from build123d import *
from OCP.BRepFilletAPI import BRepFilletAPI_MakeChamfer

# Parameters (mm, degrees)
SKETCH1_W                     = 2.54
SKETCH1_H                     = 2.54
MAIN_BODY_DEPTH               = 2.54
SKETCH3_W                     = 1.778
SKETCH3_H                     = 0.381
CUT_EXTRUDE1_DEPTH            = 5.399409051
CUT_EXTRUDE2_DEPTH            = 5.399409051
BODY_PATTERN_COUNT            = 4
BODY_PATTERN_PITCH            = 2.54
PIN_START                     = -5.54
SKETCH2_W                     = 0.64
SKETCH2_H                     = 0.64
PIN_DEPTH                     = 11.54
CHAMFER1_SIZE                 = 0.508
CHAMFER1_SIZE2                = 0.1905
CHAMFER2_SIZE                 = 0.1905
CHAMFER2_SIZE2                = 0.508
PIN_PATTERN_COUNT             = 4
PIN_PATTERN_PITCH             = 2.54
CHAMFER1_OF_PIN_PATTERN_SIZE  = 0.508
CHAMFER1_OF_PIN_PATTERN_SIZE2 = 0.1905
CHAMFER2_OF_PIN_PATTERN_SIZE2 = 0.1905
CHAMFER2_OF_PIN_PATTERN_SIZE  = 0.508


with BuildPart() as part:
    # Sketch1 → Main Body (new body)
    with BuildSketch(Plane(origin=(0, 0, 0), x_dir=(1, 0, 0), z_dir=(0, 1, 0))):
        with Locations((1.27, 1.27)):
            Rectangle(SKETCH1_W, SKETCH1_H)
    main_body = extrude(amount=MAIN_BODY_DEPTH)

    # Sketch3 → Cut-Extrude1 (cut, through all)
    with BuildSketch(Plane.ZY):
        with Locations((-1.27, 0.1905)):
            Rectangle(SKETCH3_W, SKETCH3_H)
    cut_extrude1 = extrude(amount=-CUT_EXTRUDE1_DEPTH, mode=Mode.SUBTRACT)

    # Sketch4 → Cut-Extrude2 (cut, through all)
    with BuildSketch(Plane(origin=(0, 2.54, 0), x_dir=(1, 0, 0), z_dir=(0, 1, 0))):
        Polygon((0.254, 2.54), (0, 2.54), (0, 2.032), align=None)
        Polygon((2.54, 2.54), (2.286, 2.54), (2.54, 2.032), align=None)
        Polygon((0.254, 0), (0, 0.508), (0, 0), align=None)
        Polygon((2.54, 0), (2.286, 0), (2.54, 0.508), align=None)
    cut_extrude2 = extrude(amount=-CUT_EXTRUDE2_DEPTH, mode=Mode.SUBTRACT)

    # Body Pattern: Main Body, Cut-Extrude1, Cut-Extrude2 ×4
    with Locations(*[(-i * BODY_PATTERN_PITCH, 0, 0) for i in range(1, BODY_PATTERN_COUNT)]):
        add(main_body)
        add(cut_extrude1, mode=Mode.SUBTRACT)
        add(cut_extrude2, mode=Mode.SUBTRACT)

    # Sketch2 → Pin (add)
    with BuildSketch(Plane(origin=(0, 2.54, 0), x_dir=(1, 0, 0), z_dir=(0, 1, 0)).offset(PIN_START)):
        with Locations((1.27, 1.27)):
            Rectangle(SKETCH2_W, SKETCH2_H)
    pin = extrude(amount=PIN_DEPTH)

    # Chamfer1: one chamfer whose edges measure the first distance from different faces: ONE call of the kernel's chamfer builder (chamfer() names one face for all edges)
    chamfer1_edges_1 = [part.edges().sort_by_distance(p)[0] for p in [
        (0.95, 8.54, -1.27),
    ]]
    chamfer1_side_1 = [part.faces().sort_by_distance(p)[0] for p in [
        (0.95, 5.54, -1.27),
    ]]
    chamfer1_edges_2 = [part.edges().sort_by_distance(p)[0] for p in [
        (1.27, 8.54, -0.95),
    ]]
    chamfer1_side_2 = [part.faces().sort_by_distance(p)[0] for p in [
        (1.27, 5.54, -0.95),
    ]]
    chamfer1_edges_3 = [part.edges().sort_by_distance(p)[0] for p in [
        (1.59, 8.54, -1.27),
    ]]
    chamfer1_side_3 = [part.faces().sort_by_distance(p)[0] for p in [
        (1.59, 5.54, -1.27),
    ]]
    chamfer1_edges_4 = [part.edges().sort_by_distance(p)[0] for p in [
        (1.27, 8.54, -1.59),
    ]]
    chamfer1_side_4 = [part.faces().sort_by_distance(p)[0] for p in [
        (1.27, 5.54, -1.59),
    ]]
    chamfer1 = BRepFilletAPI_MakeChamfer(part.part.solid().wrapped)
    for e in chamfer1_edges_1:
        chamfer1.Add(CHAMFER1_SIZE, CHAMFER1_SIZE2, e.wrapped, chamfer1_side_1[0].wrapped)  # the first distance lies on this face
    for e in chamfer1_edges_2:
        chamfer1.Add(CHAMFER1_SIZE, CHAMFER1_SIZE2, e.wrapped, chamfer1_side_2[0].wrapped)  # the first distance lies on this face
    for e in chamfer1_edges_3:
        chamfer1.Add(CHAMFER1_SIZE, CHAMFER1_SIZE2, e.wrapped, chamfer1_side_3[0].wrapped)  # the first distance lies on this face
    for e in chamfer1_edges_4:
        chamfer1.Add(CHAMFER1_SIZE, CHAMFER1_SIZE2, e.wrapped, chamfer1_side_4[0].wrapped)  # the first distance lies on this face
    add(Compound.cast(chamfer1.Shape()), mode=Mode.REPLACE)

    # Chamfer2
    chamfer2_edges = [part.edges().sort_by_distance(p)[0] for p in [
        (1.27, -3, -0.95),
        (1.59, -3, -1.27),
        (1.27, -3, -1.59),
        (0.95, -3, -1.27),
    ]]
    chamfer2_side = [part.faces().sort_by_distance(p)[0] for p in [
        (1.27, -3, -1.27),
    ]]
    chamfer(chamfer2_edges, length=CHAMFER2_SIZE, length2=CHAMFER2_SIZE2, reference=chamfer2_side[0])

    # Pin Pattern: Pin ×4
    with Locations(*[(-i * PIN_PATTERN_PITCH, 0, 0) for i in range(1, PIN_PATTERN_COUNT)]):
        add(pin)

    # Chamfer1 of Pin Pattern: one chamfer whose edges measure the first distance from different faces: ONE call of the kernel's chamfer builder (chamfer() names one face for all edges)
    chamfer1_of_pin_pattern_edges_1 = [part.edges().sort_by_distance(p)[0] for p in [
        (-1.59, 8.54, -1.27),
    ]]
    chamfer1_of_pin_pattern_side_1 = [part.faces().sort_by_distance(p)[0] for p in [
        (-1.59, 5.54, -1.27),
    ]]
    chamfer1_of_pin_pattern_edges_2 = [part.edges().sort_by_distance(p)[0] for p in [
        (-1.27, 8.54, -0.95),
    ]]
    chamfer1_of_pin_pattern_side_2 = [part.faces().sort_by_distance(p)[0] for p in [
        (-1.27, 5.54, -0.95),
    ]]
    chamfer1_of_pin_pattern_edges_3 = [part.edges().sort_by_distance(p)[0] for p in [
        (-0.95, 8.54, -1.27),
    ]]
    chamfer1_of_pin_pattern_side_3 = [part.faces().sort_by_distance(p)[0] for p in [
        (-0.95, 5.54, -1.27),
    ]]
    chamfer1_of_pin_pattern_edges_4 = [part.edges().sort_by_distance(p)[0] for p in [
        (-1.27, 8.54, -1.59),
    ]]
    chamfer1_of_pin_pattern_side_4 = [part.faces().sort_by_distance(p)[0] for p in [
        (-1.27, 5.54, -1.59),
    ]]
    chamfer1_of_pin_pattern_edges_5 = [part.edges().sort_by_distance(p)[0] for p in [
        (-4.13, 8.54, -1.27),
    ]]
    chamfer1_of_pin_pattern_side_5 = [part.faces().sort_by_distance(p)[0] for p in [
        (-4.13, 5.54, -1.27),
    ]]
    chamfer1_of_pin_pattern_edges_6 = [part.edges().sort_by_distance(p)[0] for p in [
        (-3.81, 8.54, -0.95),
    ]]
    chamfer1_of_pin_pattern_side_6 = [part.faces().sort_by_distance(p)[0] for p in [
        (-3.81, 5.54, -0.95),
    ]]
    chamfer1_of_pin_pattern_edges_7 = [part.edges().sort_by_distance(p)[0] for p in [
        (-3.49, 8.54, -1.27),
    ]]
    chamfer1_of_pin_pattern_side_7 = [part.faces().sort_by_distance(p)[0] for p in [
        (-3.49, 5.54, -1.27),
    ]]
    chamfer1_of_pin_pattern_edges_8 = [part.edges().sort_by_distance(p)[0] for p in [
        (-3.81, 8.54, -1.59),
    ]]
    chamfer1_of_pin_pattern_side_8 = [part.faces().sort_by_distance(p)[0] for p in [
        (-3.81, 5.54, -1.59),
    ]]
    chamfer1_of_pin_pattern_edges_9 = [part.edges().sort_by_distance(p)[0] for p in [
        (-6.67, 8.54, -1.27),
    ]]
    chamfer1_of_pin_pattern_side_9 = [part.faces().sort_by_distance(p)[0] for p in [
        (-6.67, 5.54, -1.27),
    ]]
    chamfer1_of_pin_pattern_edges_10 = [part.edges().sort_by_distance(p)[0] for p in [
        (-6.35, 8.54, -0.95),
    ]]
    chamfer1_of_pin_pattern_side_10 = [part.faces().sort_by_distance(p)[0] for p in [
        (-6.35, 5.54, -0.95),
    ]]
    chamfer1_of_pin_pattern_edges_11 = [part.edges().sort_by_distance(p)[0] for p in [
        (-6.03, 8.54, -1.27),
    ]]
    chamfer1_of_pin_pattern_side_11 = [part.faces().sort_by_distance(p)[0] for p in [
        (-6.03, 5.54, -1.27),
    ]]
    chamfer1_of_pin_pattern_edges_12 = [part.edges().sort_by_distance(p)[0] for p in [
        (-6.35, 8.54, -1.59),
    ]]
    chamfer1_of_pin_pattern_side_12 = [part.faces().sort_by_distance(p)[0] for p in [
        (-6.35, 5.54, -1.59),
    ]]
    chamfer1_of_pin_pattern = BRepFilletAPI_MakeChamfer(part.part.solid().wrapped)
    for e in chamfer1_of_pin_pattern_edges_1:
        chamfer1_of_pin_pattern.Add(CHAMFER1_OF_PIN_PATTERN_SIZE, CHAMFER1_OF_PIN_PATTERN_SIZE2, e.wrapped, chamfer1_of_pin_pattern_side_1[0].wrapped)  # the first distance lies on this face
    for e in chamfer1_of_pin_pattern_edges_2:
        chamfer1_of_pin_pattern.Add(CHAMFER1_OF_PIN_PATTERN_SIZE, CHAMFER1_OF_PIN_PATTERN_SIZE2, e.wrapped, chamfer1_of_pin_pattern_side_2[0].wrapped)  # the first distance lies on this face
    for e in chamfer1_of_pin_pattern_edges_3:
        chamfer1_of_pin_pattern.Add(CHAMFER1_OF_PIN_PATTERN_SIZE, CHAMFER1_OF_PIN_PATTERN_SIZE2, e.wrapped, chamfer1_of_pin_pattern_side_3[0].wrapped)  # the first distance lies on this face
    for e in chamfer1_of_pin_pattern_edges_4:
        chamfer1_of_pin_pattern.Add(CHAMFER1_OF_PIN_PATTERN_SIZE, CHAMFER1_OF_PIN_PATTERN_SIZE2, e.wrapped, chamfer1_of_pin_pattern_side_4[0].wrapped)  # the first distance lies on this face
    for e in chamfer1_of_pin_pattern_edges_5:
        chamfer1_of_pin_pattern.Add(CHAMFER1_OF_PIN_PATTERN_SIZE, CHAMFER1_OF_PIN_PATTERN_SIZE2, e.wrapped, chamfer1_of_pin_pattern_side_5[0].wrapped)  # the first distance lies on this face
    for e in chamfer1_of_pin_pattern_edges_6:
        chamfer1_of_pin_pattern.Add(CHAMFER1_OF_PIN_PATTERN_SIZE, CHAMFER1_OF_PIN_PATTERN_SIZE2, e.wrapped, chamfer1_of_pin_pattern_side_6[0].wrapped)  # the first distance lies on this face
    for e in chamfer1_of_pin_pattern_edges_7:
        chamfer1_of_pin_pattern.Add(CHAMFER1_OF_PIN_PATTERN_SIZE, CHAMFER1_OF_PIN_PATTERN_SIZE2, e.wrapped, chamfer1_of_pin_pattern_side_7[0].wrapped)  # the first distance lies on this face
    for e in chamfer1_of_pin_pattern_edges_8:
        chamfer1_of_pin_pattern.Add(CHAMFER1_OF_PIN_PATTERN_SIZE, CHAMFER1_OF_PIN_PATTERN_SIZE2, e.wrapped, chamfer1_of_pin_pattern_side_8[0].wrapped)  # the first distance lies on this face
    for e in chamfer1_of_pin_pattern_edges_9:
        chamfer1_of_pin_pattern.Add(CHAMFER1_OF_PIN_PATTERN_SIZE, CHAMFER1_OF_PIN_PATTERN_SIZE2, e.wrapped, chamfer1_of_pin_pattern_side_9[0].wrapped)  # the first distance lies on this face
    for e in chamfer1_of_pin_pattern_edges_10:
        chamfer1_of_pin_pattern.Add(CHAMFER1_OF_PIN_PATTERN_SIZE, CHAMFER1_OF_PIN_PATTERN_SIZE2, e.wrapped, chamfer1_of_pin_pattern_side_10[0].wrapped)  # the first distance lies on this face
    for e in chamfer1_of_pin_pattern_edges_11:
        chamfer1_of_pin_pattern.Add(CHAMFER1_OF_PIN_PATTERN_SIZE, CHAMFER1_OF_PIN_PATTERN_SIZE2, e.wrapped, chamfer1_of_pin_pattern_side_11[0].wrapped)  # the first distance lies on this face
    for e in chamfer1_of_pin_pattern_edges_12:
        chamfer1_of_pin_pattern.Add(CHAMFER1_OF_PIN_PATTERN_SIZE, CHAMFER1_OF_PIN_PATTERN_SIZE2, e.wrapped, chamfer1_of_pin_pattern_side_12[0].wrapped)  # the first distance lies on this face
    add(Compound.cast(chamfer1_of_pin_pattern.Shape()), mode=Mode.REPLACE)

    # Chamfer2 of Pin Pattern
    chamfer2_of_pin_pattern_edges = [part.edges().sort_by_distance(p)[0] for p in [
        (-1.27, -3, -0.95),
        (-0.95, -3, -1.27),
        (-1.27, -3, -1.59),
        (-1.59, -3, -1.27),
        (-3.81, -3, -0.95),
        (-3.49, -3, -1.27),
        (-3.81, -3, -1.59),
        (-4.13, -3, -1.27),
        (-6.35, -3, -0.95),
        (-6.03, -3, -1.27),
        (-6.35, -3, -1.59),
        (-6.67, -3, -1.27),
    ]]
    chamfer(chamfer2_of_pin_pattern_edges, length=CHAMFER2_OF_PIN_PATTERN_SIZE, length2=CHAMFER2_OF_PIN_PATTERN_SIZE2)


solid = part.part
Part model, mm, in its own coordinate system. Coordinates: 2 decimals unless noted, no trailing zeros. Write each loop counter-clockwise with the first axis right and the second up, starting at its lowest first coordinate (ties: lowest second). Pieces come first, ordered by that corner, then holes. Notation, with made-up numbers: M 9,-9.5 L 54,-9.5 A20 cw 54,16.5 Z; hole C -39.75,9 d4. An arc over 180 degrees is marked long. Return JSON: item names as keys, results as strings.
1. Saw through at C-C, the plane x = -5.5. Write the cut outline in (y, z).
Determined:
{"outline": "M 0,-2.54 L 2.54,-2.54 L 2.54,0 L 0,0 L 0,-0.38 L 0.38,-0.38 L 0.38,-2.16 L 0,-2.16 Z"}
2. Flat gauge pins, fed straight in: pin 1 Ø3 at (x, y) = (1.5, 5) entering from -Z; pin 2 Ø0.5 at (x, y) = (-4, 5.5) entering from +Z; pin 3 Ø1.5 at (y, z) = (-0.5, -1.5) entering from -X. Where does each tip first touch, or does it go through?
Determined:
{"pin 1": "z = -1.59", "pin 2": "z = -0.95", "pin 3": "x = -6.67"}
3. Saw through at D-D, the plane z = -2.3. Write the cut outline in (x, y).
Determined:
{"outline": "M -7.49,0 L -5.21,0 L -5.21,2.54 L -7.49,2.54 Z; M -4.95,0 L -2.67,0 L -2.67,2.54 L -4.95,2.54 Z; M -2.41,0 L -0.13,0 L -0.13,2.54 L -2.41,2.54 Z; M 0.13,0 L 2.41,0 L 2.41,2.54 L 0.13,2.54 Z"}
4. Saw through at A-A, the plane y = 5.75. Write the cut outline in (x, z).
Determined:
{"outline": "M -6.67,-1.59 L -6.03,-1.59 L -6.03,-0.95 L -6.67,-0.95 Z; M -4.13,-1.59 L -3.49,-1.59 L -3.49,-0.95 L -4.13,-0.95 Z; M -1.59,-1.59 L -0.95,-1.59 L -0.95,-0.95 L -1.59,-0.95 Z; M 0.95,-1.59 L 1.59,-1.59 L 1.59,-0.95 L 0.95,-0.95 Z"}
5. Probe L1, parallel to X at y = 3.75, z = -1.5; L2, parallel to Y at x = -7, z = -0.95. List the from-to ranges inside material, lowest first.
Determined:
{"L1": "-6.67 to -6.03, -4.13 to -3.49, -1.59 to -0.95, 0.95 to 1.59", "L2": "0.38 to 2.54"}
6. Saw through at B-B, the plane y = 1.75. Write the cut outline in (x, z), then the cut area to 3 significant figures.
Determined:
{"outline": "M -7.62,-2.03 L -7.37,-2.54 L -5.33,-2.54 L -5.08,-2.03 L -4.83,-2.54 L -2.79,-2.54 L -2.54,-2.03 L -2.29,-2.54 L -0.25,-2.54 L 0,-2.03 L 0.25,-2.54 L 2.29,-2.54 L 2.54,-2.03 L 2.54,-0.51 L 2.29,0 L 0.25,0 L 0,-0.51 L -0.25,0 L -2.29,0 L -2.54,-0.51 L -2.79,0 L -4.83,0 L -5.08,-0.51 L -5.33,0 L -7.37,0 L -7.62,-0.51 Z", "area": "24.8 mm²"}
7. Pull direction Z, two halves, no side cores. Call faces 1 (the face through (2.54, 1, -1)), 2 (the face through (-3, 0.381, -1)), 3 (the face through (1, 1, -2.54)), 4 (the face through (-1, 1, 0)): pulls with the +Z half, pulls with the -Z half, needs draft (parallel to the pull), parting line crosses it, or undercut.
Determined:
{"face 1": "needs draft", "face 2": "undercut", "face 3": "pulls with the -Z half", "face 4": "pulls with the +Z half"}
